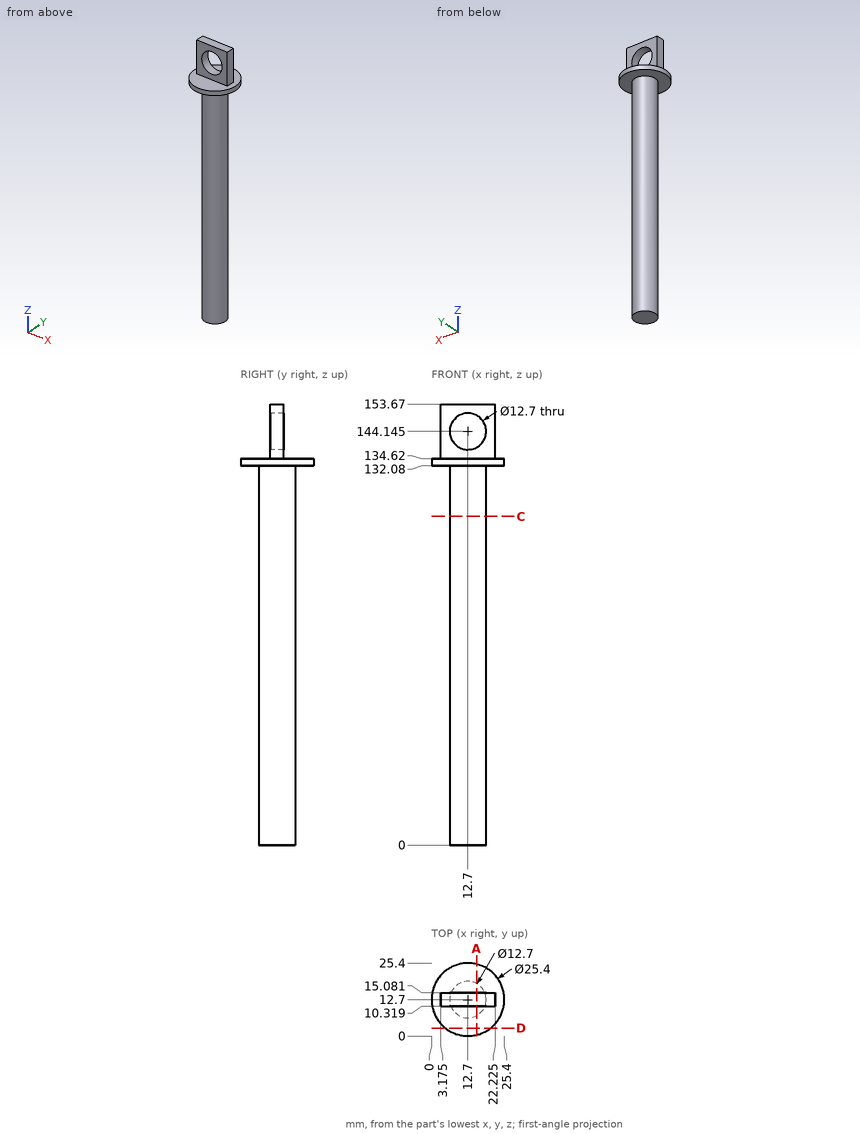
Study the drawing (mm; zero at the part's minimum x, y, z) and answer. Coordinates: 2 decimals unless noted, no trailing zeros. Order: outer loops, then holes, each group sorted by start corner. A loop starts at its lowest first (then second) coordinate and runs counter-clockwise, first axis right, second up. Notation, with made-up numbers: (34, 87.25) -> (58, 87.25) arc R34 ccw to (58, 119.25) -> close; hole circle Ø3 at (-12.5, 12). An arc over 180 degrees is marked (long way). Answer in a Markdown table with one row per item. Add a question column.
Item 1: Find section C-C (z = 114.5). Write down the section's boundary in (x, y), then the cut area to 3 significant figures.
Item 2: Find section A-A (x = 15.75). Write down the section's boundary in (y, z) (1 decimal), then the cut area to 3 significant figures.
Item 3: Each of these flat-tipped pins is pushed along its axis until it touches: P1, Ø5, axis at x = 8, z = 136.5, coming from the -Y side; P2, Ø2.5, axis at y = 13.5, z = 146.5, coming from the +X side (3 decimals); P3, Ø2, axis at x = 8, y = 18.5, coming from the +Z side; P4, Ø11.5, axis at x = 12.7, z = 144.145, coming from the -Y side (3 decimals). Where does it stop, or does it pass through?
Item 4: Find section D-D (y = 2.75). Write down the section's boundary in (x, z).
Item 5: Find the intervals of material crossed by L1, parallel to Z at x = 12.7, y = 14.1 (1 decimal); L2, parallel to Z at x = 8.25, y = 3.5; L3, parallel to Z at x = 11.25, y = 15.5, in increasing order. Write a range as from..to.
Result set:
| question | item | result |
|---|---|---|
| 1 | outline | circle Ø12.7 at (12.7, 12.7) |
| 1 | area | 127 mm² |
| 2 | outline | (0.4, 132.1) -> (7.1, 132.1) -> (7.1, 0) -> (18.3, 0) -> (18.3, 132.1) -> (25, 132.1) -> (25, 134.6) -> (15.1, 134.6) -> (15.1, 138.6) -> (10.3, 138.6) -> (10.3, 134.6) -> (0.4, 134.6) -> close; (10.3, 149.7) -> (15.1, 149.7) -> (15.1, 153.7) -> (10.3, 153.7) -> close |
| 2 | area | 1,570 mm² |
| 3 | P1 | stops at y = 0.37 |
| 3 | P2 | stops at x = 22.225 |
| 3 | P3 | stops at z = 134.62 |
| 3 | P4 | passes through |
| 4 | outline | (4.81, 132.08) -> (20.59, 132.08) -> (20.59, 134.62) -> (4.81, 134.62) -> close |
| 5 | L1 | z = 0..137.8, 150.5..153.7 |
| 5 | L2 | z = 132.08..134.62 |
| 5 | L3 | z = 0..134.62 |
